Drawing for the job (mm, zero at the part's lowest x, y, z). A direction names the side the tool comes from. Round coordinates to 2 decimals unless told otherwise and drop trailing zeros. Loops run counter-clockwise (first coordinate to the right, second up) from the corner with the lowest first, then second, coordinate; pieces in that order, holes last. Notation, with made-up numbers: M -34.75,-36 L 12.25,-36 A8 ccw 12.25,-30 Z; hole C 33,53 d10. An arc over 180 degrees is marked long. Answer in a Markdown table with one row per item.
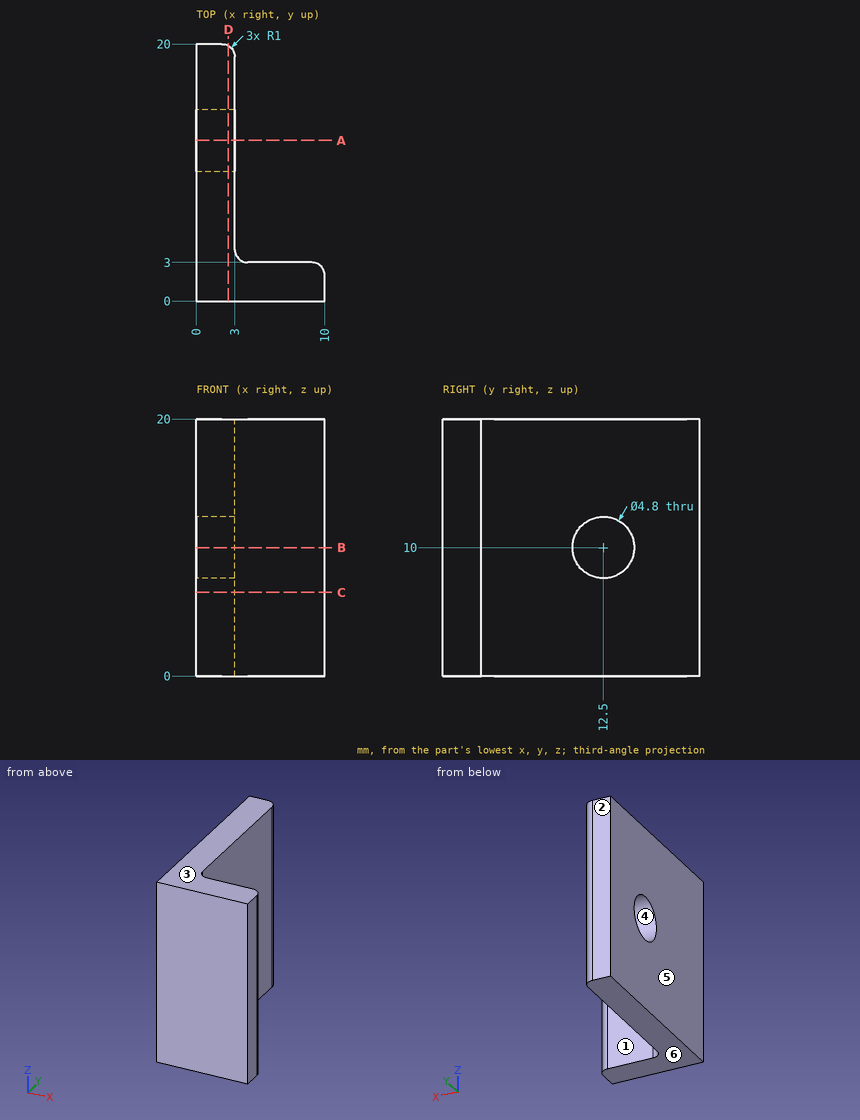
1. Pin check, flat tips, straight feed: pin 1 (5.5 mm diameter, centred on y = 12.5, z = 10, fed in from -X); pin 2 (2 mm diameter, centred on y = 13, z = 5, fed in from +X); pin 3 (2.5 mm diameter, centred on x = 7, z = 6.5, fed in from +Y). Stop position of each tip, or through.
Verdict:
| item | result |
|---|---|
| pin 1 | stops at x = 0 |
| pin 2 | stops at x = 3 |
| pin 3 | stops at y = 3 |
2. Saw through at C-C (z = 6.5). Write the cut outline in (x, y).
Verdict:
| item | result |
|---|---|
| outline | M 0,0 L 10,0 L 10,2 A1 ccw 9,3 L 4,3 A1 cw 3,4 L 3,19 A1 ccw 2,20 L 0,20 Z |
3. Mould opens along Z. For the marked faces 3, 4, 5 and 6 say: +Z half, -Z half, draft (parallel to the pull), parting line (faces both ways), or undercut.
Verdict:
| item | result |
|---|---|
| face 3 | +Z half |
| face 4 | undercut |
| face 5 | draft |
| face 6 | -Z half |
4. Saw through at A-A (y = 12.5). Write the cut outline in (x, z), and give its area (3 significant figures).
Verdict:
| item | result |
|---|---|
| outline | M 0,0 L 3,0 L 3,7.6 L 0,7.6 Z; M 0,12.4 L 3,12.4 L 3,20 L 0,20 Z |
| area | 45.6 mm² |
5. Saw through at B-B (z = 10). Write the cut outline in (x, y).
Verdict:
| item | result |
|---|---|
| outline | M 0,0 L 10,0 L 10,2 A1 ccw 9,3 L 4,3 A1 cw 3,4 L 3,10.1 L 0,10.1 Z; M 0,14.9 L 3,14.9 L 3,19 A1 ccw 2,20 L 0,20 Z |
6. Saw through at D-D (x = 2.5). Write the cut outline in (y, z), and give its area (3 significant figures).
Verdict:
| item | result |
|---|---|
| outline | M 0,0 L 19.87,0 L 19.87,20 L 0,20 Z; hole C 12.5,10 d4.8 |
| area | 379 mm² |
7. Wall check: probe 1 along Y at (x, z) = (6.75, 11); probe 2 along Z at (x, y) = (1.6, 12.5). Give the ranges that are in metal, low to high.
Verdict:
| item | result |
|---|---|
| probe 1 | y = 0 to 3 |
| probe 2 | z = 0 to 7.6, 12.4 to 20 |
8. Tool access for the marked faces 1 and 2: list every direction of +Z, -Z, +X, -X, +Y, -Y with a clear straight run to the whole face (end or side of a thin tool).
Verdict:
| item | result |
|---|---|
| face 1 | +Z, -Z, +X, +Y |
| face 2 | +Z, -Z, +X, -X, +Y |
